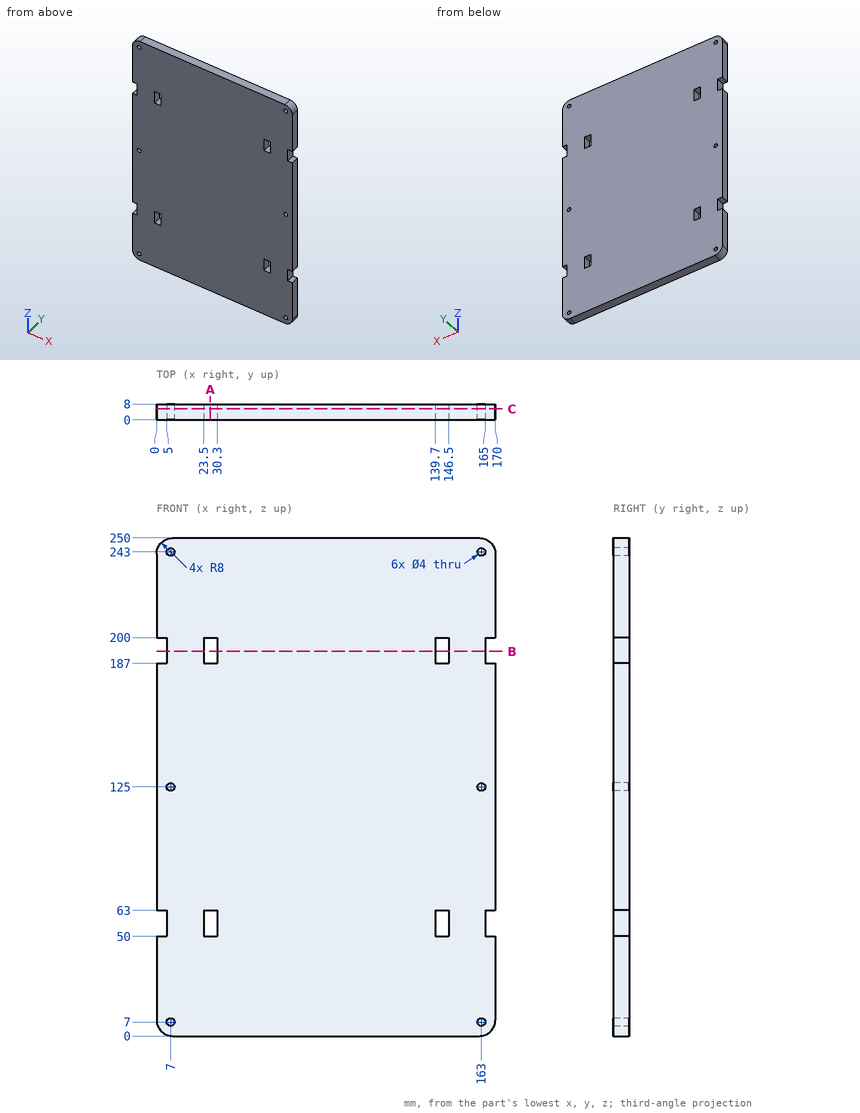
Answer from the drawing. Dimensions are ordinates in mm from the lowest x, y and z of the part. Round coordinates to 2 decimals unless told otherwise and drop trailing zeros. Loops run counter-clockwise (first coordinate to the right, second up) from the corner with the lowest first, then second, coordinate; pieces in that order, holes last.
1) Given P1, Ø4, axis at y = 3, z = 194, coming from the +X side; P2, Ø2.5, axis at x = 7, z = 7, coming from the -Y side; P3, Ø2.5, axis at x = 2, y = 3.5, coming from the +Z side, each flat-ended and moving along its own axis, determine where each tip first touches the part or whether it passes through.
Outcome:
P1: stops at x = 165
P2: passes through
P3: stops at z = 248.44
2) A cutting plane is placed at A-A on x = 27. Determine the outline of the cut face in (y, z), plus the area to 3 significant figures.
Outcome:
outline: (0, 0) - (8, 0) - (8, 50) - (0, 50) - close; (0, 63) - (8, 63) - (8, 187) - (0, 187) - close; (0, 200) - (8, 200) - (8, 250) - (0, 250) - close
area: 1,790 mm2
3) A cutting plane is placed at C-C on y = 5.5. Give the number of separate pieces and of enclosed holes in the cut face, plus the area to 3 significant figures.
Outcome:
separate pieces: 1
enclosed holes: 10
area: 41,800 mm2
4) Consider line 1 (X direction, y = 0.5, z = 195.5); line 2 (X direction, y = 5.5, z = 125); line 3 (Z direction, x = 163, y = 5). Determine where each line is inside the solid, lowest interval first.
Outcome:
line 1: x = 5 to 23.5, 30.3 to 139.7, 146.5 to 165
line 2: x = 0 to 5, 9 to 161, 165 to 170
line 3: z = 0.06 to 5, 9 to 123, 127 to 241, 245 to 249.94
5) A cutting plane is placed at B-B on z = 193. Determine the outline of the cut face in (x, y), plus the area to 3 significant figures.
Outcome:
outline: (5, 0) - (23.5, 0) - (23.5, 8) - (5, 8) - close; (30.3, 0) - (139.7, 0) - (139.7, 8) - (30.3, 8) - close; (146.5, 0) - (165, 0) - (165, 8) - (146.5, 8) - close
area: 1,170 mm2
